For this review, take the finished solid that the model builds, in its own axes (mm). Face numbers are marked on the shaded views. Round coordinates to 2 decimals unless told otherwise and drop trailing zeros. Write each loop counter-clockwise with the first axis right and the second up, starting at its lowest first coordinate (ties: lowest second). Pieces come first, ordered by that corner, then holes. Notation, with made-up numbers: M 44.5,81.5 L 83.5,81.5 A15 ccw 83.5,87.5 Z; hole C -30,-25.5 d1. An arc over 180 degrees is marked long. Use one line per item in the form item = value. Start each with the question number.
Item 1: Add section B-B (z = 0). State the section outline as (x, y) points.
Item 2: For line 1 (Z direction, x = 3, y = 45.5); line 2 (Y direction, x = -11, z = -13.5); line 3 (X direction, y = 77, z = -8.5), list the stretches that pass through material, from the lowest coordinate up. Write a range as [from, to].
Item 3: Add section C-C (x = 2). State the section outline as (y, z) points, and give its area (3 significant figures).
Item 4: Add section D-D (z = 13). State the section outline as (x, y) points.
Item 5: Draft analysis for pull direction Z (two halves, no side actions). For the marked faces 1, 2 and 3, state which applies: released by +Z, released by -Z, zero draft, split by the parting line, or undercut.
Item 6: Add section A-A (y = 19). State the section outline as (x, z) points, and give its area (3 significant figures).
Item 7: For P1, Ø5, axis at y = 73.5, z = 4, coming from the -X side; P2, Ø5, axis at x = 6, y = 38.5, coming from the -Z side; P3, Ø14.5, axis at x = -9.5, y = 67, coming from the +Z side; P4, Ø5, axis at y = 46.5, z = 4, coming from the -X side, all flat-tipped, find the tip position at first contact; note any pin that passes through.
from build123d import *

# Parameters (mm, degrees)
CROQUIS2_R              = 17.5
SALIENTE_EXTRUIR1_DEPTH = 2
CROQUIS3_R              = 15.5
SALIENTE_EXTRUIR2_DEPTH = 10
CROQUIS6_W              = 20
CROQUIS6_H              = 5
SALIENTE_EXTRUIR4_DEPTH = 80
CROQUIS7_R              = 2
CORTAR_EXTRUIR4_DEPTH   = 97.577783797
REDONDEO1_R             = 3


with BuildPart() as part:
    # Croquis2 → Saliente-Extruir1 (new body)
    with BuildSketch(Plane(origin=(0, 0, 0), x_dir=(1, 0, 0), z_dir=(0, 1, 0))):
        with Locations(Location((0, 0, 0), (0, 0, 270))):
            Circle(CROQUIS2_R)
    extrude(amount=SALIENTE_EXTRUIR1_DEPTH)

    # Croquis3 → Saliente-Extruir2 (add)
    with BuildSketch(Plane(origin=(0, 2, 0), x_dir=(1, 0, 0), z_dir=(0, 1, 0))):
        with Locations(Location((0, 0, 0), (0, 0, 270))):
            Circle(CROQUIS3_R)
    extrude(amount=SALIENTE_EXTRUIR2_DEPTH)

    # Cortar con superficie2
    split(bisect_by=Plane(origin=(-1.264952602, 9.000605443, 0), x_dir=(0, 0, 1), z_dir=(-0.13917310096006574, 0.9902680687415703, 0)), keep=Keep.BOTTOM)

    # Croquis6 → Saliente-Extruir4 (add)
    with BuildSketch(Plane(origin=(-1.264952602, 9.000605443, 0), x_dir=(0.9902680687415704, 0.13917310096006577, 0), z_dir=(-0.13917310096006577, 0.9902680687415704, 0))):
        with Locations((0.7, -8.5)):
            Rectangle(CROQUIS6_W, CROQUIS6_H)
    saliente_extruir4 = extrude(amount=SALIENTE_EXTRUIR4_DEPTH)

    # Croquis7 → Cortar-Extruir4 (cut, through all)
    with BuildSketch(Plane.XY.offset(11)):
        with BuildLine():
            Line((-21.608293718, 86.927741104), (-19.938216506, 75.044524279))
            add(Edge.make_bspline(
                [(-19.938216506, 75.044524279), (-16.656953462, 87.623606273), (-11.705613295, 88.319472076)],
                knots=[0, 0, 0, 0.499999987, 0.499999987, 0.499999987], degree=2))
            Line((-11.705613295, 88.319472076), (-21.608293718, 86.927741104))
        make_face()
        with BuildLine():
            Line((-1.802932343, 89.711203123), (-11.705613295, 88.319472076))
            add(Edge.make_bspline(
                [(-11.705613295, 88.319472076), (-6.754272863, 89.015337917), (-0.132855132, 77.827986298)],
                knots=[0.499999987, 0.499999987, 0.499999987, 1, 1, 1], degree=2))
            Line((-0.132855132, 77.827986298), (-1.802932343, 89.711203123))
        make_face()
        with Locations((-10.300204683, 78.319472113)):
            Circle(CROQUIS7_R)
    cortar_extruir4 = extrude(amount=-CORTAR_EXTRUIR4_DEPTH, mode=Mode.SUBTRACT)

    # Simetría1: Saliente-Extruir4, Cortar-Extruir4 across plane
    add(saliente_extruir4.mirror(Plane.XY))
    add(cortar_extruir4.mirror(Plane.XY), mode=Mode.SUBTRACT)

    # Redondeo1
    redondeo1_edges = [part.edges().sort_by_distance(p)[0] for p in [
        (-0.132855132, 77.827986298, 8.5),
        (-19.938216506, 75.044524279, 8.5),
        (-0.132855132, 77.827986298, -8.5),
        (-19.938216506, 75.044524279, -8.5),
    ]]
    fillet(redondeo1_edges, radius=REDONDEO1_R)


solid = part.part
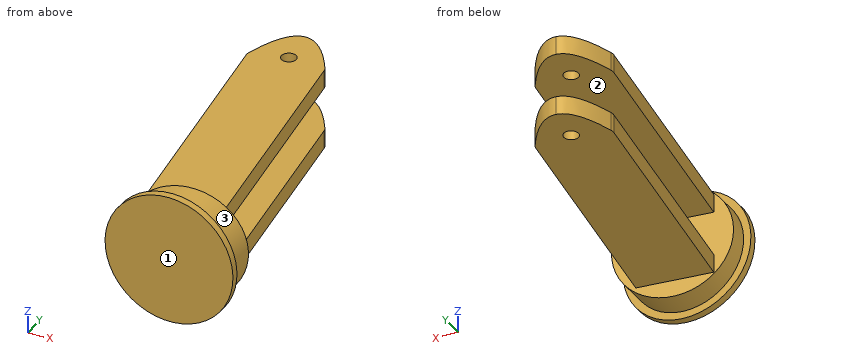
Calculated:
q1.outline = M -17.5,0 L 17.5,0 L 17.5,2 L 15.5,2 L 15.5,11.36 L -15.5,7 L -15.5,2 L -17.5,2 Z
q2.line_1 = [-11, -6], [6, 11]
q2.line_2 = [0, 2]
q2.line_3 = [-19.4, -11.8], [-8.8, -0.02]
q3.outline = M 0,-17.39 L 2,-17.39 L 2,-15.37 L 9.46,-15.37 L 9.46,-11 L 62.65,-11 L 62.65,-6 L 9.46,-6 L 9.46,6 L 62.65,6 L 62.65,11 L 9.46,11 L 9.46,15.37 L 2,15.37 L 2,17.39 L 0,17.39 Z
q3.area = 831 mm^2
q4.outline = M -11.72,0 L 11.72,0 L 11.72,2 L 8.44,2 L 8.44,10.36 L -8.44,7.99 L -8.44,2 L -11.72,2 Z
q5.face_1 = zero draft
q5.face_2 = undercut
q5.face_3 = split by the parting line
q6.outline = M -12.06,-11 L 8.13,-11 L 8.13,-6 L -12.06,-6 Z; M -12.06,6 L 8.13,6 L 8.13,11 L -12.06,11 Z
q6.area = 202 mm^2
q7.P1 = -19.88
q7.P2 = -11
q7.P3 = 11
q7.P4 = -16.14
